The figure shows three views and two pictorial views of one solid part (mm, origin at its lowest corner). Answer the questions. Give positions to 0.01 mm unless a question says otherwise; leave off trailing zeros. Loops run counter-clockwise (first coordinate to the right, second up) from the corner with the lowest first, then second, coordinate; pieces in that order, holes last. Notation, with made-up numbers: (-3.75, 14.5) - (48.25, 14.5) arc R20 ccw to (48.25, 29.5) - close; hole circle Ø5 at (5.25, 70). An arc over 180 degrees is marked (long way). Use CSV: the item, a comma, the result in double quotes.
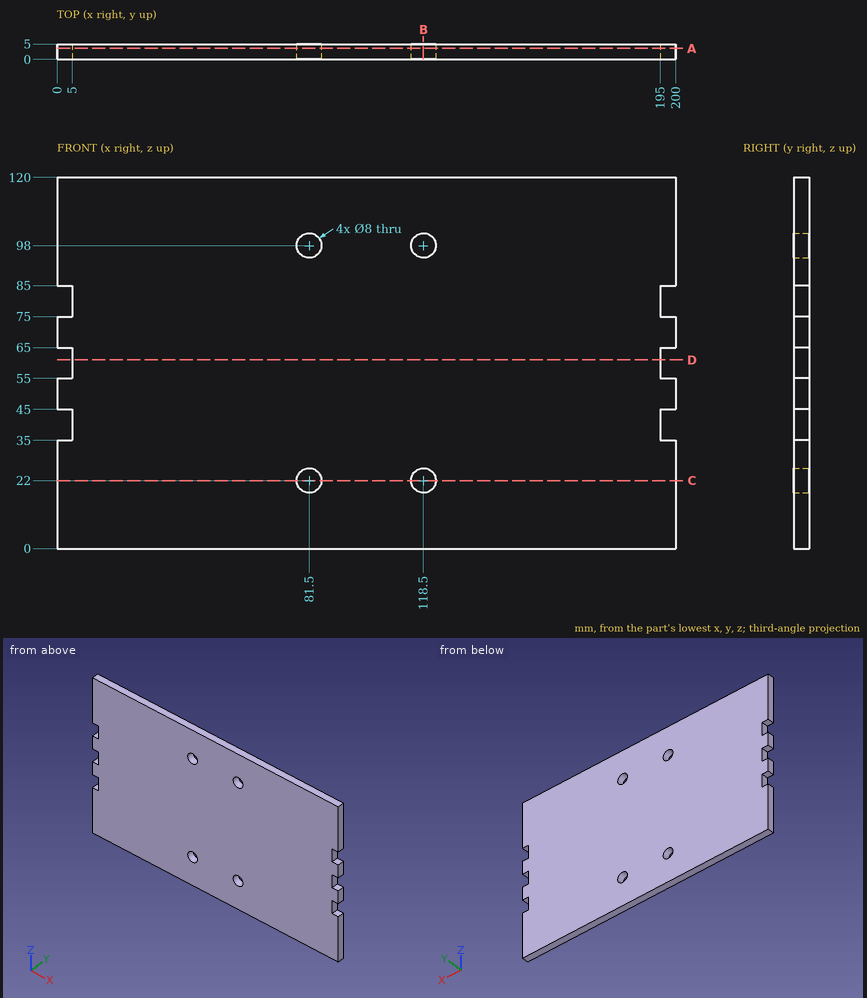
Item 1: Given P1, Ø2.5, axis at y = 2.5, z = 60.5, coming from the +X side; P2, Ø2.5, axis at y = 3.5, z = 42, coming from the -X side; P3, Ø6.5, axis at x = 118.5, z = 22, coming from the -Y side, each flat-ended and moving along its own axis, determine where each tip first touches the part or whether it passes through.
Determined:
P1,"stops at x = 195"
P2,"stops at x = 5"
P3,"passes through"
Item 2: A cutting plane is placed at B-B on x = 118.5. Determine the outline of the cut face in (y, z).
Determined:
outline,"(0, 0) - (5, 0) - (5, 18) - (0, 18) - close; (0, 26) - (5, 26) - (5, 94) - (0, 94) - close; (0, 102) - (5, 102) - (5, 120) - (0, 120) - close"
Item 3: A cutting plane is placed at D-D on z = 61. Determine the outline of the cut face in (x, y).
Determined:
outline,"(5, 0) - (195, 0) - (195, 5) - (5, 5) - close"
Item 4: A cutting plane is placed at C-C on z = 22. Determine the outline of the cut face in (x, y).
Determined:
outline,"(0, 0) - (77.5, 0) - (77.5, 5) - (0, 5) - close; (85.5, 0) - (114.5, 0) - (114.5, 5) - (85.5, 5) - close; (122.5, 0) - (200, 0) - (200, 5) - (122.5, 5) - close"
Item 5: Find the intervals of material crossed by line 1 (X direction, y = 3.25, z = 98); line 2 (Z direction, x = 118.5, y = 2.15); line 3 (Z direction, x = 82.5, y = 3.15), in increasing order.
Determined:
line 1,"x = 0 to 77.5, 85.5 to 114.5, 122.5 to 200"
line 2,"z = 0 to 18, 26 to 94, 102 to 120"
line 3,"z = 0 to 18.13, 25.87 to 94.13, 101.87 to 120"
Item 6: A cutting plane is placed at A-A on y = 3.6. State how many separate pieces and enclosed holes the cut face has, and give its area (3 significant figures).
Determined:
separate pieces,"1"
enclosed holes,"4"
area,"23,500 mm²"
